Could you check a few things on this model? Use its own coordinates, in mm. A direction names the side the tool comes from. Round coordinates to 2 decimals unless told otherwise and drop trailing zeros. Order: outer loops, then holes, each group sorted by start corner. A loop starts at its lowest first (then second) coordinate and runs counter-clockwise, first axis right, second up.
Autodesk Inventor part; units mm, degrees
ref_plane "HGO_ANBAU_XY" through (0, 0, 0) normal (0, 1, 0) x (1, 0, 0)
ref_plane "HGO_ANBAU_YZ" through (0, 0, 0) normal (1, 0, 0) x (0, 0, -1)
ref_plane "HGO_ANBAU_ZX" through (0, 0, 0) normal (0, 0, -1) x (0, 1, 0)
sketch "Sketch_4" plane through (0, 0, 0) normal (0, 0, 1) x (1, 0, 0)
  line L0 (-6, 12) -> (-6, 0)
  line L1 (-6, 0) -> (6, 0)
  line L2 (6, 0) -> (6, 12)
  line L3 (6, 12) -> (-6, 12)
extrude "Extrusion1" add sketch "Sketch_4" along normal mid plane 52
sketch "Sketch2" plane through (-6, 12, 26) normal (0, 1, 0) x (1, 0, 0)
  point P0 (6, 46)
hole "Hole1" at (0, 12, -20) direction (0, -1, 0) diameter 5.5 depth 12 counterbore diameter 10 counterbore depth 5.8
sketch "Sketch3" plane through (-6, 12, 26) normal (0, 1, 0) x (1, 0, 0)
  point P0 (6, 6)
hole "Hole2" at (0, 12, 20) direction (0, -1, 0) diameter 5.5 depth 12 counterbore diameter 10 counterbore depth 5.8
sketch "Sketch_13" plane through (0, 0, 0) normal (1, 0, 0) x (0, 0, -1)
  line L0 (10, 0) -> (10, 12)
  line L1 (10, 12) -> (12.5, 12)
  line L2 (12.5, 12) -> (12.067, 11.567)
  line L3 (12.067, 11.567) -> (12.067, 0.433)
  line L4 (12.067, 0.433) -> (12.5, 0)
  line L5 (12.5, 0) -> (10, 0)
  line L6 (10, 0) -> (10, 12)
revolve "Revolution1" cut sketch "Sketch_13" angle 360 about axis through (0, 0, -10) along (0, -1, 0)
thread "Thread1"
sketch "Sketch_14" plane through (0, 0, 0) normal (1, 0, 0) x (0, 0, -1)
  line L0 (-10, 0) -> (-10, 12)
  line L1 (-10, 12) -> (-7.5, 12)
  line L2 (-7.5, 12) -> (-7.933, 11.567)
  line L3 (-7.933, 11.567) -> (-7.933, 0.433)
  line L4 (-7.933, 0.433) -> (-7.5, 0)
  line L5 (-7.5, 0) -> (-10, 0)
  line L6 (-10, 0) -> (-10, 12)
revolve "Revolution2" cut sketch "Sketch_14" angle 360 about axis through (0, 0, 10) along (0, -1, 0)
thread "Thread2"
sketch "Sketch6" plane through (-6, 0, 26) normal (0, -1, 0) x (1, 0, 0)
  point P0 (4, -26)
hole "Hole3" at (-2, 0, 0) direction (0, 1, 0) diameter 5 depth 12
ref_plane "HGO_ANBAU_XY" through (0, 0, 0) normal (0, 1, 0) x (1, 0, 0)
ref_plane "HGO_ANBAU_YZ" through (0, 0, 0) normal (1, 0, 0) x (0, 0, -1)
ref_plane "HGO_ANBAU_ZX" through (0, 0, 0) normal (0, 0, -1) x (0, 1, 0)
ref_plane "HGO_ANBAU_Schrauben_1_XY" through (0, 5.5, -20) normal (0, -1, 0) x (1, 0, 0)
ref_plane "HGO_ANBAU_Schrauben_1_YZ" through (0, 5.5, -20) normal (1, 0, 0) x (0, 0, 1)
ref_plane "HGO_ANBAU_Schrauben_1_ZX" through (0, 5.5, -20) normal (0, 0, 1) x (0, -1, 0)
ref_plane "HGO_ANBAU_Schrauben_2_XY" through (0, 5.5, 20) normal (0, -1, 0) x (1, 0, 0)
ref_plane "HGO_ANBAU_Schrauben_2_YZ" through (0, 5.5, 20) normal (1, 0, 0) x (0, 0, 1)
ref_plane "HGO_ANBAU_Schrauben_2_ZX" through (0, 5.5, 20) normal (0, 0, 1) x (0, -1, 0)
ref_plane "KLEMMHALTER_XY" through (0, 12, 0) normal (0, 1, 0) x (1, 0, 0)
ref_plane "KLEMMHALTER_YZ" through (0, 12, 0) normal (1, 0, 0) x (0, 0, -1)
ref_plane "KLEMMHALTER_ZX" through (0, 12, 0) normal (0, 0, -1) x (0, 1, 0)
properties part number "722627 MUE-70/80P2"
Q1. Imagine slicing it at B-B, the plane x = -4. Please give me the cut outline in (y, z), then the cut area to 3 significant figures.
Q2. Imagine slicing it at D-D, the plane z = 0. Please give me the cut outline in (x, y).
Q3. We'd pull the mould along X, two halves only. Please class faces 1 (the cylindrical face through (-0.121, 3.057, -22.747)), 2 (the flat face through (-6, 6, 0)), 3 (the flat face through (1, 0, 0)): released by +X, released by -X, zero draft, split by the parting line, or undercut.
Q4. Imagine slicing it at C-C, the plane y = 4.25. Please give me the cut outline in (x, z).
Q5. Imagine slicing it at A-A, the plane z = -10. Please give me the cut outline in (x, y), then the cut area to 3 significant figures.
Q6. I need wall thicknesses on L1, parallel to X at y = 5.75, z = 0; L2, parallel to Z at x = -1.5, y = 0.75; L3, parallel to Z at x = -3.5, y = 9. Which ranges of each line are inside material? Lowest first, please.
Q7. For faces 4 (the cylindrical face through (0, 9, -25)), 5 (the cylindrical face through (0.091, 5.922, -7.935)), which set-ups out of +Z, -Z, +X, -X, +Y, -Y let a thin tool reach every point of the face, with its end or its side?
Q8. For P1, Ø3, axis at x = 1, z = -21.5, coming from the +Y side, with a flat end and sliding along its axis, tell me the tip position at first contact or that it passes through.
Filled in:
1. outline: (0, -26) - (12, -26) - (12, -23) - (6.2, -23) - (6.2, -17) - (12, -17) - (12, -1.5) - (0, -1.5) - close; (0, 1.5) - (12, 1.5) - (12, 17) - (6.2, 17) - (6.2, 23) - (12, 23) - (12, 26) - (0, 26) - close
1. area: 518 mm2
2. outline: (-6, 0) - (-4.5, 0) - (-4.5, 12) - (-6, 12) - close; (0.5, 0) - (6, 0) - (6, 12) - (0.5, 12) - close
3. face 1: undercut
3. face 2: released by -X
3. face 3: zero draft
4. outline: (-6, -26) - (6, -26) - (6, 26) - (-6, 26) - close; hole circle Ø5 at (-2, 0); hole circle Ø5.5 at (0, -20); hole circle Ø5.5 at (0, 20); hole circle Ø4.13 at (0, -10); hole circle Ø4.13 at (0, 10)
5. outline: (-6, 0) - (-2.5, 0) - (-2.07, 0.43) - (-2.07, 11.57) - (-2.5, 12) - (-6, 12) - close; (2.07, 0.43) - (2.5, 0) - (6, 0) - (6, 12) - (2.5, 12) - (2.07, 11.57) - close
5. area: 94.0 mm2
6. L1: x = -6 to -4.5, 0.5 to 6
6. L2: z = -26 to -22.3, -17.7 to -11.42, -8.58 to -2.45, 2.45 to 8.58, 11.42 to 17.7, 22.3 to 26
6. L3: z = -26 to -23.57, -16.43 to -2, 2 to 16.43, 23.57 to 26
7. face 4: +Y
7. face 5: +Y, -Y
8. P1: stops at y = 6.2
